The figure shows three views and two pictorial views of one solid part (mm, origin at its lowest corner). Answer the questions. Coordinates: 2 decimals unless noted, no trailing zeros. Loops run counter-clockwise (first coordinate to the right, second up) from the corner with the lowest first, then second, coordinate; pieces in that order, holes last. Notation, with made-up numbers: (3.25, 57) -> (38.25, 57) arc R27 cw to (38.25, 90) -> close; hole circle Ø3 at (70.25, 33.5). An arc over 180 degrees is marked (long way). Answer in a Markdown table with one row per item.
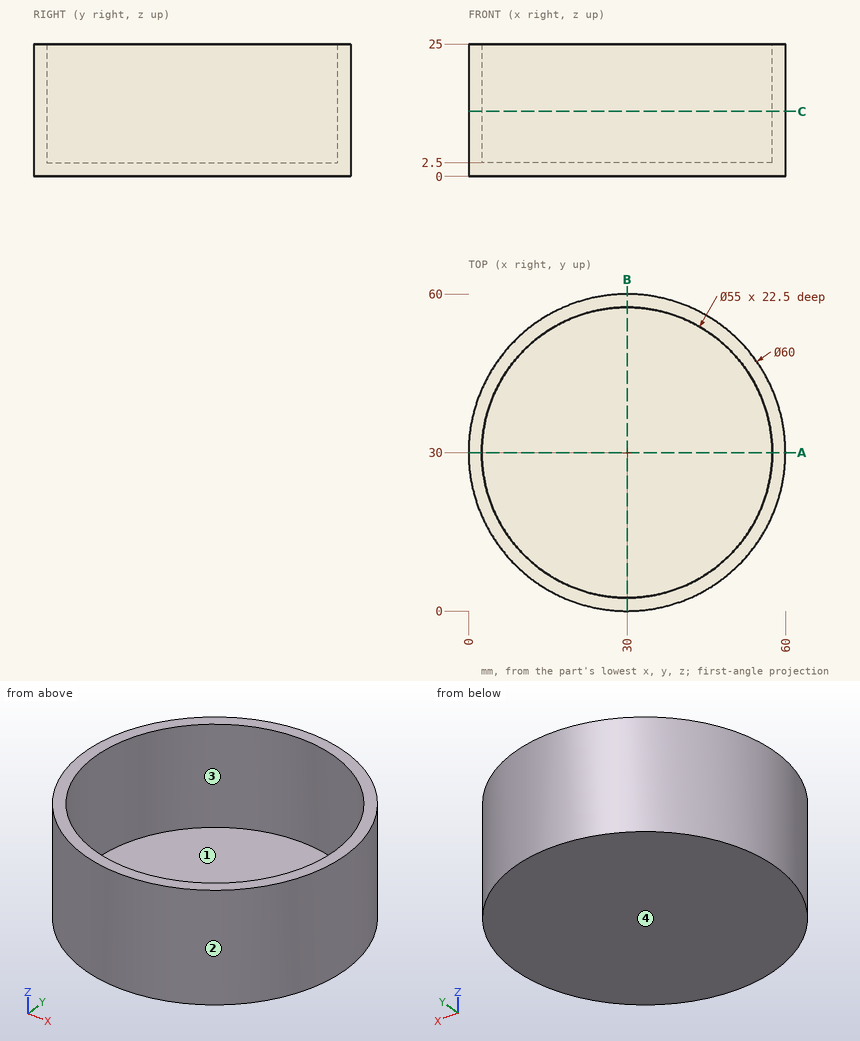
Item 1: A cutting plane is placed at A-A, the plane y = 30. Determine the outline of the cut face in (x, z), plus the area to 4 significant figures.
Findings below:
| item | result |
|---|---|
| outline | (0, 0) -> (60, 0) -> (60, 25) -> (57.5, 25) -> (57.5, 2.5) -> (2.5, 2.5) -> (2.5, 25) -> (0, 25) -> close |
| area | 262.5 mm2 |
Item 2: Determine the mould class of the marked faces 1, 2, 3 and 4 for opening direction Y: +Y half, -Y half, draft (parallel to the pull), parting line (faces both ways), or undercut.
Findings below:
| item | result |
|---|---|
| face 1 | undercut |
| face 2 | parting line |
| face 3 | undercut |
| face 4 | draft |
Item 3: A cutting plane is placed at C-C, the plane z = 12.25. Determine the outline of the cut face in (x, y).
Findings below:
| item | result |
|---|---|
| outline | circle Ø60 at (30, 30); hole circle Ø55 at (30, 30) |
Item 4: Find the intervals of material crossed by probe 1 along Y at (x, z) = (30, 20.5); probe 2 along Z at (x, y) = (21, 28.5); probe 3 along Y at (x, z) = (8.5, 13.5), in increasing order.
Findings below:
| item | result |
|---|---|
| probe 1 | y = 0 to 2.5, 57.5 to 60 |
| probe 2 | z = 0 to 2.5 |
| probe 3 | y = 9.08 to 12.85, 47.15 to 50.92 |
Item 5: Flat-ended cylindrical pins translate along their axes: pin 1 Ø1 at (y, z) = (40, 21) entering from +X; pin 2 Ø6 at (x, y) = (34.5, 39.5) entering from +Z; pin 3 Ø2 at (y, z) = (12.5, 5.5) entering from +X. Find the tip coordinate at first contact, or state that the pin passes through.
Findings below:
| item | result |
|---|---|
| pin 1 | stops at x = 58.46 |
| pin 2 | stops at z = 2.5 |
| pin 3 | stops at x = 55.05 |
